Could you check a few things on this model? Use its own coordinates, in mm. Face numbers are marked on the shaded views. A direction names the side the tool comes from. Give positions to 0.01 mm unless a question says otherwise; leave off trailing zeros. Loops run counter-clockwise (first coordinate to the right, second up) from the corner with the lowest first, then second, coordinate; pieces in that order, holes last. Notation, with made-up numbers: M 22,54.25 L 51,54.25 A8 ccw 51,59.25 Z; hole C 28,22.25 d7. An arc over 180 degrees is marked long. Return JSON: item names as keys, results as strings. Group by question number.
1. Please list where these lines run through material, in increasing order: line 1 (Y direction, x = 47, z = 5.5); line 2 (X direction, y = 12.5, z = 8.75); line 3 (X direction, y = 15, z = 5.5).
2. If we section it at A-A (z = 4.25): State how many separate pieces and enclosed holes the cut face has, plus the area to 3 significant figures.
3. For the marked faces 4 and 5, which set-ups out of +Z, -Z, +X, -X, +Y, -Y let a thin tool reach every point of the face, with its end or its side?
4. If we section it at C-C (x = 41.5): Write out the boundary of the cut face in (y, z).
5. For pin 1 (14 mm diameter, centred on x = 21, y = 10.5, fed in from +Z); pin 2 (1.5 mm diameter, centred on x = 3.5, y = -3.5, fed in from +Z), each with a flat end and sliding along its axis, tell me the tip position at first contact or that it passes through.
6. If we section it at B-B (y = 6.5): Write out the boundary of the cut face in (x, z).
7. If we mould it in two halves opening along Y, with no side actions, what happens to the marked faces 1, 2 and 3? For each: +Y half, -Y half, draft (parallel to the pull), parting line (faces both ways), or undercut.
8. If we section it at D-D (y = 15): Write out the boundary of the cut face in (x, z).
```python
from build123d import *

# Parameters (mm, degrees)
F0_W     = 58
F0_H     = 36
F0_R     = 1.25
F0_R_2   = 1.5
F1_DEPTH = 10
F0_R_3   = 1
F0_W_2   = 3.2825097442
F0_H_2   = 9.0816104785
F2_DEPTH = 2.5
F3_R     = 3
F4_DEPTH = 6
F5_START = 0.9
F5_DEPTH = 16.2
F6_START = 6
F6_DEPTH = 10.7
F7_R     = 1


with BuildPart() as f1:
    # F0 (on Top) → F1 (new body)
    with BuildSketch(Plane.XY):
        with Locations((22.1260370687, 12.181818096)):
            Rectangle(F0_W, F0_H)
        with Locations((-2.8739629313, -1.818181904)):
            Circle(F0_R, mode=Mode.SUBTRACT)
        with Locations((3.1260370687, -3.018181904)):
            Circle(F0_R_2, mode=Mode.SUBTRACT)
        with Locations((41.1260370687, -3.018181904)):
            Circle(F0_R_2, mode=Mode.SUBTRACT)
        with Locations((47.1260370687, -1.818181904)):
            Circle(F0_R, mode=Mode.SUBTRACT)
        with BuildLine():
            Line((-0.0042433119, 0.0237876128), (-0.0123524841, 0.02397218))
            Line((-0.0123524841, 0.02397218), (-0.0123524841, 0.0693824727))
            ThreePointArc((-0.0123524841, 0.0693824727), (-1.0671188126, 12.0466773263), (-0.0123524841, 24.02397218))
            ThreePointArc((-0.0123524841, 24.02397218), (22.4498159336, 26.0118318189), (44.9770614896, 25))
            ThreePointArc((44.9770614896, 25), (46.474513746, 12), (44.9770614896, -1))
            ThreePointArc((44.9770614896, -1), (22.4574664967, -1.8971785964), (0, 0))
            ThreePointArc((0, 0), (-0.0021227043, 0.0118936194), (-0.0042433119, 0.0237876128))
        make_face(mode=Mode.SUBTRACT)
        with Locations((-2.8739629313, 26.181818096)):
            Circle(F0_R, mode=Mode.SUBTRACT)
        with Locations((3.1260370687, 27.16396598)):
            Circle(F0_R_2, mode=Mode.SUBTRACT)
        with Locations((41.1260370687, 27.6376707083)):
            Circle(F0_R_2, mode=Mode.SUBTRACT)
        with Locations((47.1260370687, 26.181818096)):
            Circle(F0_R, mode=Mode.SUBTRACT)
        with Locations((-2.8739629313, 26.181818096)):
            Circle(F0_R)
        with Locations((47.1260370687, 26.181818096)):
            Circle(F0_R)
        with Locations((47.1260370687, -1.818181904)):
            Circle(F0_R)
        with Locations((-2.8739629313, -1.818181904)):
            Circle(F0_R)
        with Locations((3.1260370687, -3.018181904)):
            Circle(F0_R_2)
        with Locations((3.1260370687, 27.16396598)):
            Circle(F0_R_2)
        with Locations((41.1260370687, 27.6376707083)):
            Circle(F0_R_2)
        with Locations((41.1260370687, -3.018181904)):
            Circle(F0_R_2)
    extrude(amount=F1_DEPTH)

    # F0 (on Top) → F2 (join)
    with BuildSketch(Plane.XY):
        with BuildLine():
            ThreePointArc((-0.0123524841, 24.02397218), (-1.0671188126, 12.0466773263), (-0.0123524841, 0.0693824727))
            Line((-0.0123524841, 0.0693824727), (-0.0123524841, 24.02397218))
        make_face()
        with BuildLine():
            Line((-0.0123524841, 24.02397218), (-0.0123524841, 0.0693824727))
            ThreePointArc((-0.0123524841, 0.0693824727), (-0.0083017494, 0.0465843578), (-0.0042433119, 0.0237876128))
            Line((-0.0042433119, 0.0237876128), (44.9770614896, -1))
            Line((44.9770614896, -1), (44.9770614896, 25))
            Line((44.9770614896, 25), (-0.0123524841, 24.02397218))
        make_face()
        with Locations((2.9621722015, 2.0848012064)):
            Circle(F0_R_3, mode=Mode.SUBTRACT)
        with Locations((5.0146379508, 11.9371688925)):
            Rectangle(F0_W_2, F0_H_2, mode=Mode.SUBTRACT)
        with Locations((41.7125664489, 2.0848012064)):
            Circle(F0_R_3, mode=Mode.SUBTRACT)
        with BuildLine():
            Line((26.1260370687, 7.1930042468), (26.1260370687, 9.181818096))
            Line((26.1260370687, 9.181818096), (26.4652403515, 9.181818096))
            ThreePointArc((26.4652403515, 9.181818096), (32.1260370687, 13.1930042468), (37.7868337859, 9.181818096))
            Line((37.7868337859, 9.181818096), (38.1260370687, 9.181818096))
            Line((38.1260370687, 9.181818096), (38.1260370687, 7.1930042468))
            Line((38.1260370687, 7.1930042468), (38.1260370687, 1.181818096))
            Line((38.1260370687, 1.181818096), (26.1260370687, 1.181818096))
            Line((26.1260370687, 1.181818096), (26.1260370687, 7.1930042468))
        make_face(mode=Mode.SUBTRACT)
        with Locations((41.1260370687, 12.181818096)):
            Circle(F0_R_2, mode=Mode.SUBTRACT)
        with Locations((18.8074270263, 12.2937392443)):
            Circle(F0_R_3, mode=Mode.SUBTRACT)
        with Locations((2.9621722015, 21.6664075851)):
            Circle(F0_R_3, mode=Mode.SUBTRACT)
        with Locations((26.8074270263, 12.2937392443)):
            Circle(F0_R_3, mode=Mode.SUBTRACT)
        with Locations((41.7125664489, 21.6664075851)):
            Circle(F0_R_3, mode=Mode.SUBTRACT)
        with BuildLine():
            Line((44.9770614896, -1), (-0.0042433119, 0.0237876128))
            ThreePointArc((-0.0042433119, 0.0237876128), (-0.0021227043, 0.0118936194), (0, 0))
            ThreePointArc((0, 0), (22.4574664967, -1.8971785964), (44.9770614896, -1))
        make_face()
        with BuildLine():
            ThreePointArc((44.9770614896, 25), (22.4498159336, 26.0118318189), (-0.0123524841, 24.02397218))
            Line((-0.0123524841, 24.02397218), (44.9770614896, 25))
        make_face()
        with BuildLine():
            Line((44.9770614896, 25), (44.9770614896, -1))
            ThreePointArc((44.9770614896, -1), (46.474513746, 12), (44.9770614896, 25))
        make_face()
        with Locations((2.9621722015, 21.6664075851)):
            Circle(F0_R_3)
        with Locations((2.9621722015, 2.0848012064)):
            Circle(F0_R_3)
        with Locations((41.7125664489, 2.0848012064)):
            Circle(F0_R_3)
        with Locations((41.7125664489, 21.6664075851)):
            Circle(F0_R_3)
        with Locations((18.8074270263, 12.2937392443)):
            Circle(F0_R_3)
        with Locations((26.8074270263, 12.2937392443)):
            Circle(F0_R_3)
        with Locations((5.0146379508, 11.9371688925)):
            Rectangle(F0_W_2, F0_H_2)
        with BuildLine():
            Line((26.4652403515, 9.181818096), (26.1260370687, 9.181818096))
            Line((26.1260370687, 9.181818096), (26.1260370687, 7.1930042468))
            ThreePointArc((26.1260370687, 7.1930042468), (26.2114457767, 8.2017707453), (26.4652403515, 9.181818096))
        make_face()
        with BuildLine():
            ThreePointArc((38.1260370687, 7.1930042468), (32.1260370687, 1.1930042468), (26.1260370687, 7.1930042468))
            Line((26.1260370687, 7.1930042468), (26.1260370687, 1.181818096))
            Line((26.1260370687, 1.181818096), (38.1260370687, 1.181818096))
            Line((38.1260370687, 1.181818096), (38.1260370687, 7.1930042468))
        make_face()
        with BuildLine():
            Line((38.1260370687, 9.181818096), (37.7868337859, 9.181818096))
            ThreePointArc((37.7868337859, 9.181818096), (38.0406283607, 8.2017707453), (38.1260370687, 7.1930042468))
            Line((38.1260370687, 7.1930042468), (38.1260370687, 9.181818096))
        make_face()
    extrude(amount=F2_DEPTH)

    # F3
    f3_edges = [f1.edges().sort_by_distance(p)[0] for p in [
        (51.126037, 30.181818, 5),
        (51.126037, -5.818182, 5),
        (-6.873963, -5.818182, 5),
        (-6.873963, 30.181818, 5),
    ]]
    fillet(f3_edges, radius=F3_R)

    # F0 (on Top) → F4 (join)
    with BuildSketch(Plane.XY):
        with Locations((5.0146379508, 11.9371688925)):
            Rectangle(F0_W_2, F0_H_2)
    extrude(amount=F4_DEPTH)

    # F0 (on Top) → F5 (cut)
    with BuildSketch(Plane.XY.offset(F5_START)):
        with Locations((47.1260370687, 26.181818096)):
            Circle(F0_R)
        with Locations((-2.8739629313, 26.181818096)):
            Circle(F0_R)
        with Locations((-2.8739629313, -1.818181904)):
            Circle(F0_R)
        with Locations((47.1260370687, -1.818181904)):
            Circle(F0_R)
    extrude(amount=F5_DEPTH, mode=Mode.SUBTRACT)

    # F0 (on Top) → F6 (cut)
    with BuildSketch(Plane.XY.offset(F6_START)):
        with Locations((3.1260370687, 27.16396598)):
            Circle(F0_R_2)
        with Locations((41.1260370687, 27.6376707083)):
            Circle(F0_R_2)
        with Locations((41.1260370687, -3.018181904)):
            Circle(F0_R_2)
        with Locations((3.1260370687, -3.018181904)):
            Circle(F0_R_2)
    extrude(amount=F6_DEPTH, mode=Mode.SUBTRACT)

    # F7
    f7_edges = [f1.edges().sort_by_distance(p)[0] for p in [
        (51.126037, 12.181818, 0),
        (22.126037, -5.818182, 0),
        (50.247357, -4.939502, 0),
        (50.247357, 29.303138, 0),
        (22.126037, 30.181818, 0),
        (-5.995283, 29.303138, 0),
        (-6.873963, 12.181818, 0),
        (-5.995283, -4.939502, 0),
    ]]
    fillet(f7_edges, radius=F7_R)


solid = f1.part
```
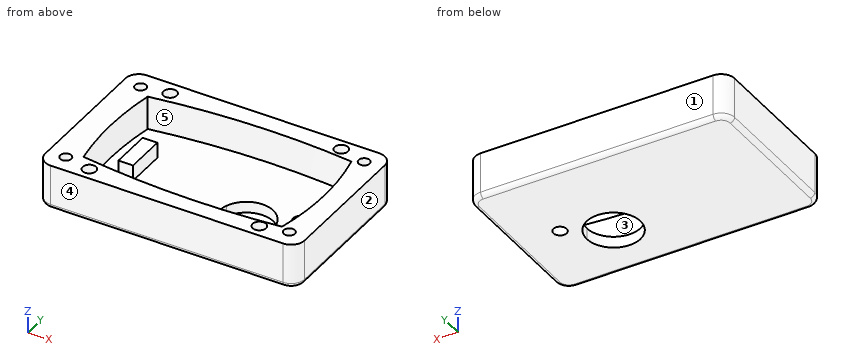
Answer:
{
 "1": {"line 1": "y = -5.82 to -3.06, -0.57 to 24.94, 27.43 to 30.18", "line 2": "x = -6.87 to -1.07, 46.47 to 51.13", "line 3": "x = -6.87 to -1, 3.37 to 6.66, 46.4 to 51.13"},
 "2": {"separate pieces": "2", "enclosed holes": "5", "area": "835 mm²"},
 "3": {"face 4": "+Z, -Z, +X, -X, -Y", "face 5": "+Z"},
 "4": {"outline": "M -5.82,1 A1 ccw -4.82,0 L 10.73,0 L 10.73,2.5 L -1.32,2.5 L -1.32,10 L -1.57,10 L -1.57,6 L -4.47,6 L -4.47,10 L -5.82,10 Z; M 13.63,0 L 29.18,0 A1 ccw 30.18,1 L 30.18,10 L 29.09,10 L 29.09,6 L 26.19,6 L 26.19,10 L 25.35,10 L 25.35,2.5 L 13.63,2.5 Z"},
 "5": {"pin 1": "stops at z = 2.5", "pin 2": "stops at z = 6"},
 "6": {"outline": "M -6.87,1 A1 ccw -5.87,0 L 26.17,0 L 26.17,2.5 L -0.84,2.5 L -0.84,10 L -6.87,10 Z; M 38.09,0 L 50.13,0 A1 ccw 51.13,1 L 51.13,10 L 46.21,10 L 46.21,2.5 L 38.09,2.5 Z"},
 "7": {"face 1": "+Y half", "face 2": "draft", "face 3": "undercut"},
 "8": {"outline": "M -6.87,1 A1 ccw -5.87,0 L 50.13,0 A1 ccw 51.13,1 L 51.13,10 L 46.4,10 L 46.4,2.5 L 6.66,2.5 L 6.66,6 L 3.37,6 L 3.37,2.5 L -1,2.5 L -1,10 L -6.87,10 Z"}
}
